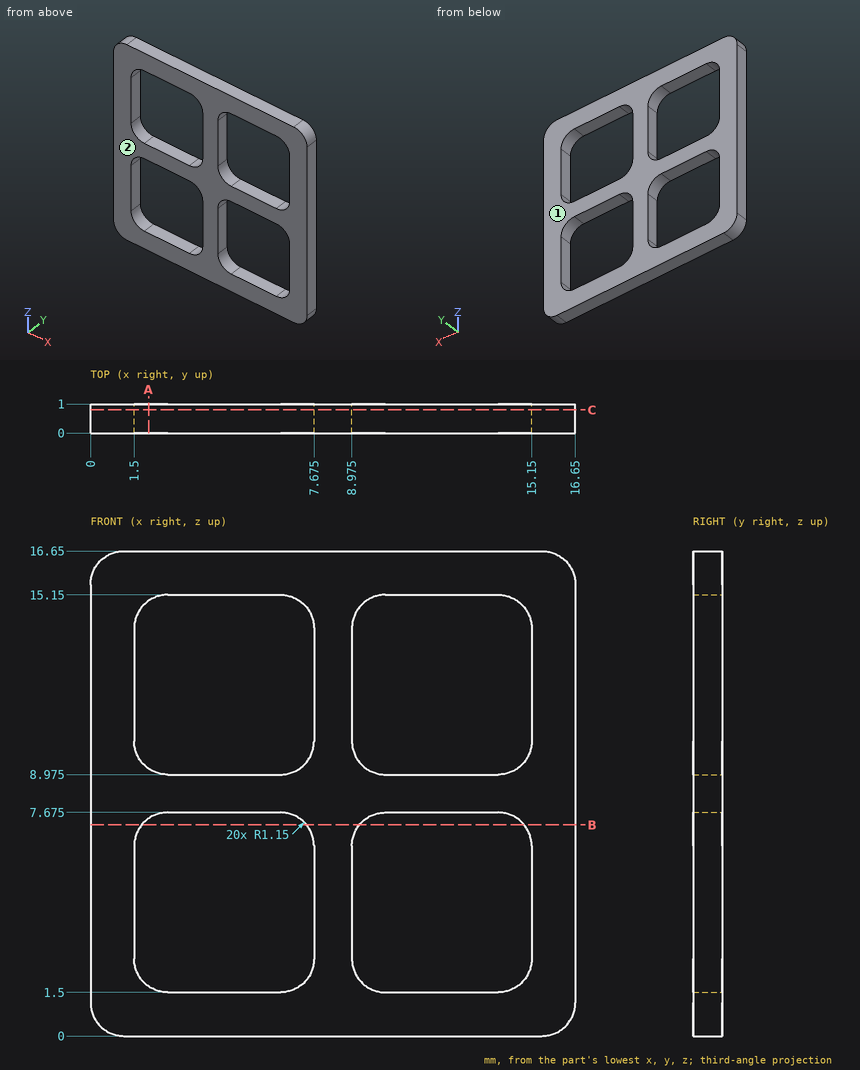
Job drawing, mm, ordinate dimensions from the low corner. One solid piece. Round coordinates to 2 decimals unless told otherwise and drop trailing zeros. Order: outer loops, then holes, each group sorted by start corner. A loop starts at its lowest first (then second) coordinate and runs counter-clockwise, first axis right, second up. Notation, with made-up numbers: (77.5, 85.25) -> (95.5, 85.25) arc R36 cw to (95.5, 120.25) -> close; hole circle Ø9 at (30.25, 84.25). An arc over 180 degrees is marked (long way). Write item = value, one per line.
(1) Pull direction Y, two halves, no side cores. Call the marked faces 1 and 2: +Y half, -Y half, draft (parallel to the pull), parting line (faces both ways), or undercut.
Answers follow:
face_1 = +Y half
face_2 = -Y half
(2) Drill centre line: L1, parallel to X at y = 0.9, z = 13.75 (3 decimals). Where is it in solid material? Low to high.
Answers follow:
L1 = 0 to 1.5, 7.675 to 8.975, 15.15 to 16.65
(3) Cut at B-B (z = 7.25). Write the cut outline in (x, y), plus the area to 3 significant figures.
Answers follow:
outline = (0, 0) -> (1.76, 0) -> (1.76, 1) -> (0, 1) -> close; (7.42, 0) -> (9.23, 0) -> (9.23, 1) -> (7.42, 1) -> close; (14.89, 0) -> (16.65, 0) -> (16.65, 1) -> (14.89, 1) -> close
area = 5.33 mm²
(4) Flat gauge pin, fed straight in: P1, Ø2, axis at x = 12, z = 1.5, coming from the -Y side. Where does the tip first touch, or does it go through?
Answers follow:
P1 = 0
(5) Cut at A-A (x = 2). Write the cut outline in (y, z), plus the area to 3 significant figures.
Answers follow:
outline = (0, 0) -> (1, 0) -> (1, 1.7) -> (0, 1.7) -> close; (0, 7.47) -> (1, 7.47) -> (1, 9.18) -> (0, 9.18) -> close; (0, 14.95) -> (1, 14.95) -> (1, 16.65) -> (0, 16.65) -> close
area = 5.11 mm²
(6) Cut at C-C (y = 0.8). State how many separate pieces and enclosed holes the cut face has, plus the area to 3 significant figures.
Answers follow:
separate_pieces = 1
enclosed_holes = 4
area = 128 mm²
